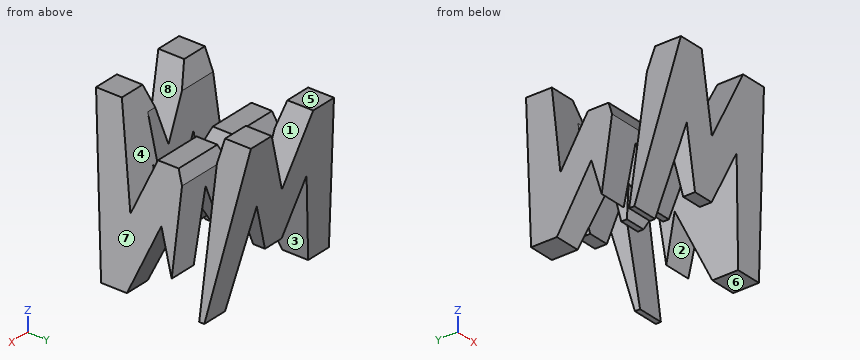
```python
from build123d import *

# Parameters (mm, degrees)
F0_W      = 38.1
F0_H      = 38.1
F1_DEPTH  = 38.1
F6_DEPTH  = 38.1
F8_DEPTH  = 38.1
F9_W      = 25.4
F9_H      = 7.62
F10_DEPTH = 38.1


with BuildPart() as f1:
    # F0 (on Front) → F1 (new body)
    with BuildSketch(Plane.XZ):
        with Locations((19.05, 19.05)):
            Rectangle(F0_W, F0_H)
    extrude(amount=F1_DEPTH)

    # F5 (on offset) → F6 (cut)
    with BuildSketch(Plane.YZ.offset(38.1)):
        Polygon((-11.43, 15.875), (-6.35, 38.1), (-31.75, 38.1), (-26.67, 15.875), (-21.59, 28.575), (-16.51, 28.575), align=None)
        Polygon((-38.1, 0), (-31.75, 0), (-38.1, 38.1), align=None)
        Polygon((-25.4, 0), (-12.7, 0), (-19.05, 15.875), align=None)
        Polygon((-6.35, 0), (0, 0), (0, 38.1), align=None)
    extrude(amount=-F6_DEPTH, mode=Mode.SUBTRACT)

    # F7 (on offset) → F8 (cut)
    with BuildSketch(Plane.XZ.offset(38.1)):
        Polygon((0, 38.1), (0, 0), (6.35, 38.1), align=None)
        Polygon((25.4, 38.1), (12.7, 38.1), (19.05, 22.555536744), align=None)
        Polygon((31.75, 38.1), (38.1, 0), (38.1, 38.1), align=None)
        Polygon((11.43, 22.225), (6.35, 0), (31.75, 0), (26.67, 22.225), (21.59, 9.855536744), (16.51, 9.855536744), align=None)
    extrude(amount=-F8_DEPTH, mode=Mode.SUBTRACT)

    # F9 (on offset) → F10 (cut)
    with BuildSketch(Plane.XY.offset(38.1)):
        with Locations((25.4, -11.43)):
            Rectangle(F9_W, F9_H)
        with Locations((12.7, -26.67)):
            Rectangle(F9_W, F9_H)
    extrude(amount=-F10_DEPTH, mode=Mode.SUBTRACT)


solid = f1.part
```
Check sheet for the modelled part. Datum: model origin and axes. Units: mm. Face numbers are marked on the shaded views. A direction names the side the tool comes from. Give positions to 0.01 mm unless a question says otherwise; leave off trailing zeros. Write each loop counter-clockwise with the first axis right and the second up, starting at its lowest first coordinate (ties: lowest second). Pieces come first, ordered by that corner, then holes.
Item 1: Access from +Z, -Z, +X, -X, +Y, -Y to the whole of each face (thin tool, end or side, straight path). Record for the marked faces 1, 2, 3, 4 and 5.
Item 2: Draft check along X on the marked faces 6, 7 and 8. Enter one of: released by +X, released by -X, zero draft, split by the parting line, or undercut.
Item 3: Gauge pin test, flat ends, axial feed: pin 1 (0.9 mm diameter, centred on x = 18.5, y = -32.5, fed in from -Z); pin 2 (2 mm diameter, centred on y = -24.5, z = 21, fed in from -X); pin 3 (9.5 mm diameter, centred on x = 23, z = 15.5, fed in from +Y) (3 decimals). Record the tip position at first contact, or that the pin passes through.
Item 4: Scan lines: L1, parallel to Y at x = 31, z = 19; L2, parallel to X at y = -34, z = 14; L3, parallel to Y at x = 29.5, z = 11.5. Record each from-to range of solid material in increasing order.
Item 5: Cross-section at A-A (z = 23.5). Count the separate pieces of the cut face and the enclosed holes in it, and give its area (3 significant figures).
Item 6: Cross-section at D-D (x = 12). Enter the section's corners in (y, z) (3 decimals), and give its area (3 significant figures).
Report:
1. face 1: +Z, +Y, -Y
1. face 2: -Z, +X, -X
1. face 3: -Z, +Y, -Y
1. face 4: +Z, +X, -X
1. face 5: +Z, +X, -X, +Y, -Y
2. face 6: zero draft
2. face 7: released by +X
2. face 8: undercut
3. pin 1: stops at z = 9.86
3. pin 2: stops at x = 25.4
3. pin 3: stops at y = -2.975
4. L1: y = -34.92 to -27.38, -25.42 to -15.24, -7.62 to -3.18
4. L2: x = 2.33 to 9.55, 14.81 to 23.29, 28.55 to 35.77
4. L3: y = -33.67 to -20.8, -17.3 to -15.24, -7.62 to -4.43
5. separate pieces: 6
5. enclosed holes: 0
5. area: 580 mm2
6. outline: (-38.1, 38.1) - (-35.223, 20.837) - (-30.48, 20.837) - (-30.48, 32.544) - (-31.75, 38.1) - close; (-22.86, 20.837) - (-13.415, 20.837) - (-16.51, 28.575) - (-21.59, 28.575) - (-22.86, 25.4) - close; (-10.296, 20.837) - (-2.877, 20.837) - (0, 38.1) - (-6.35, 38.1) - close
6. area: 281 mm2
